Study the drawing (mm; zero at the part's minimum x, y, z) and answer. A direction names the side the tool comes from. Round coordinates to 2 decimals unless told otherwise and drop trailing zeros. Loops run counter-clockwise (first coordinate to the right, second up) from the corner with the lowest first, then second, coordinate; pieces in that order, holes last. Notation, with made-up numbers: (-7.75, -26.5) - (41.25, -26.5) arc R18 ccw to (41.25, -12.5) - close; hole circle Ø5 at (22, 44). An arc over 180 degrees is marked (long way). Use CSV: the item, a comma, the result in double quotes. Start each with the question number.
1. A tool of negligible diameter and unlimited length cuts with its end or side. For the marked faces 1, 2 and 3, from which of +Z, -Z, +X, -X, +Y, -Y can it reach the whole face along a straight path? Write none if from no direction.
2. Find section D-D (y = 12). Give the vertices of the cut face in (x, z).
3. Given pin 1 Ø2.5 at (y, z) = (5, 3.5) entering from -X; pin 2 Ø0.9 at (x, y) = (28, 4.5) entering from +Z; pin 3 Ø12 at (x, y) = (23, 14.5) entering from -Z; pin 4 Ø4 at (x, z) = (16, 4) entering from -Y, each flat-ended and moving along its own axis, determine where each tip first touches the part or whether it passes through.
4. Find section C-C (x = 10.5). Give the vertices of the cut face in (y, z) (1 decimal).
5. Find section B-B (x = 25). Give the vertices of the cut face in (y, z).
6. Find section A-A (y = 4). Give the vertices of the cut face in (x, z).
7. Consider line 1 along Y through (x, z) = (9, 1.5); line 2 along Z through (x, y) = (4.5, 11); line 3 along Y through (x, z) = (11.5, 5.75). Determine where each line is inside the solid, lowest interval first.
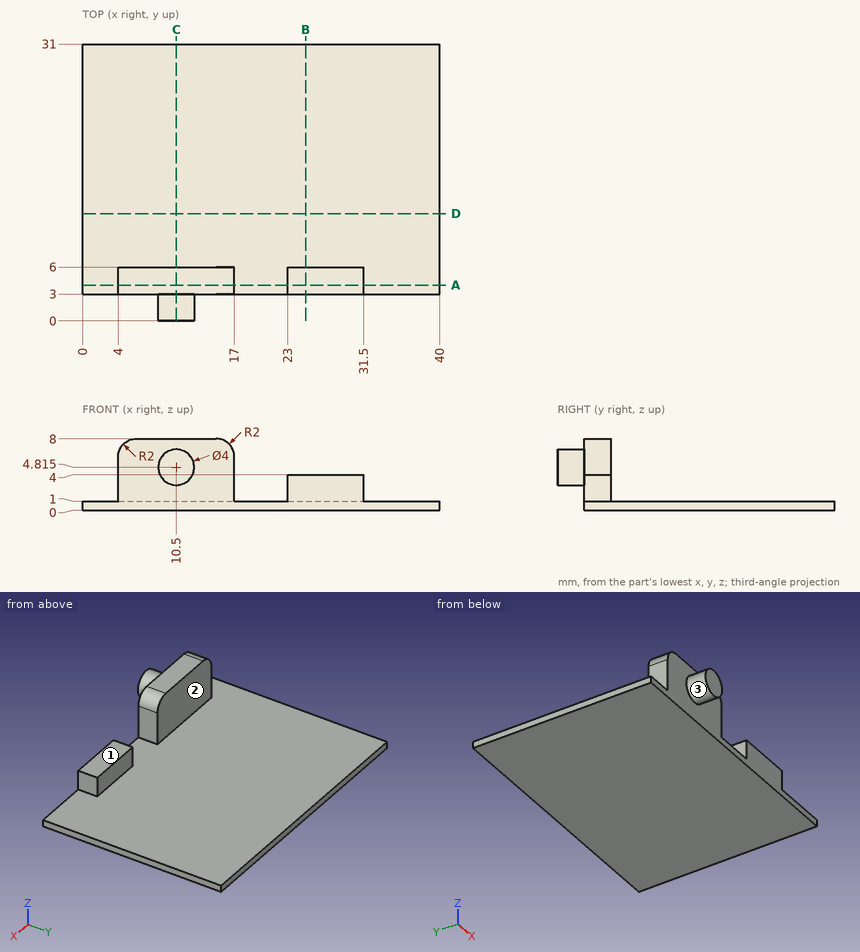
Filled sheet:
1,face 1,"+Z, +X, +Y, -Y"
1,face 2,"+Z, +X, -X, +Y"
1,face 3,"-Y"
2,outline,"(0, 0) - (40, 0) - (40, 1) - (0, 1) - close"
3,pin 1,"stops at x = 4"
3,pin 2,"stops at z = 4"
3,pin 3,"stops at z = 0"
3,pin 4,"stops at y = 3"
4,outline,"(0, 2.8) - (3, 2.8) - (3, 0) - (31, 0) - (31, 1) - (6, 1) - (6, 8) - (3, 8) - (3, 6.8) - (0, 6.8) - close"
5,outline,"(3, 0) - (31, 0) - (31, 1) - (6, 1) - (6, 4) - (3, 4) - close"
6,outline,"(0, 0) - (40, 0) - (40, 1) - (31.5, 1) - (31.5, 4) - (23, 4) - (23, 1) - (17, 1) - (17, 6) arc R2 ccw to (15, 8) - (6, 8) arc R2 ccw to (4, 6) - (4, 1) - (0, 1) - close"
7,line 1,"y = 3 to 6"
7,line 2,"z = 0 to 1"
7,line 3,"y = 0 to 6"
